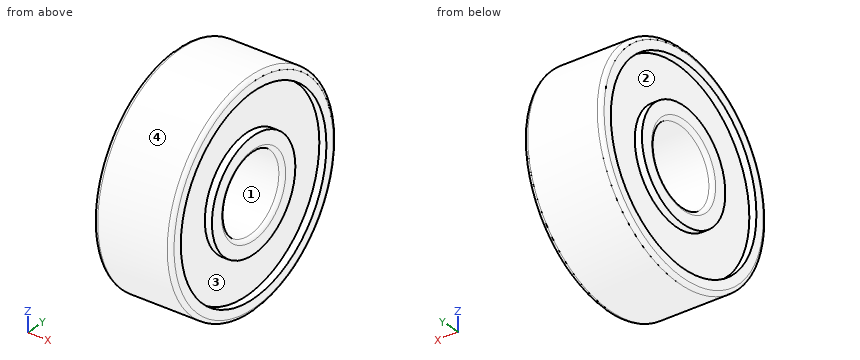
from build123d import *

# Parameters (mm, degrees)
FILLET1_R = 0.3


with BuildPart() as part:
    # Sketch1 → Revolve1 (revolve)
    with BuildSketch(Plane.XY):
        Polygon((0, 3), (6, 3), (6, 4.3), (5.45, 4.3), (5.45, 7.5), (6, 7.5), (6, 8.5), (0, 8.5), (0, 7.5), (0.55, 7.5), (0.55, 4.3), (0, 4.3), align=None)
    revolve(axis=Axis((0, 0, 0), (1, 0, 0)))

    # Fillet1
    fillet1_edges = [part.edges().sort_by_distance(p)[0] for p in [
        (0, -8.5, 0),
        (6, -8.5, 0),
        (6, -3, 0),
        (0, -3, 0),
    ]]
    fillet(fillet1_edges, radius=FILLET1_R)


solid = part.part
CAD build for the part. Positions are in the model's coordinates, mm. Face numbers are marked on the shaded views. A direction names the side the tool comes from. Give positions to 0.01 mm unless a question says otherwise; leave off trailing zeros. Write each loop counter-clockwise with the first axis right and the second up, starting at its lowest first coordinate (ties: lowest second). Pieces come first, ordered by that corner, then holes. Notation, with made-up numbers: (42.5, -37.5) -> (88.5, -37.5) arc R12 cw to (88.5, -18.5) -> close; hole circle Ø11 at (29, 55). An arc over 180 degrees is marked (long way). Return JSON: item names as keys, results as strings.
Item 1: Tool access for the marked faces 1 and 2: list every direction of +Z, -Z, +X, -X, +Y, -Y with a clear straight run to the whole face (end or side of a thin tool).
Answer below:
{"face 1": "+X, -X", "face 2": "-X"}
Item 2: Drill centre lines: probe 1 along Z at (x, y) = (5.6, 0); probe 2 along Z at (x, y) = (2.6, 0); probe 3 along Y at (x, z) = (5.5, 2). Where is each one in solid material? Low to high.
Answer below:
{"probe 1": "z = -8.5 to -7.5, -4.3 to -3, 3 to 4.3, 7.5 to 8.5", "probe 2": "z = -8.5 to -3, 3 to 8.5", "probe 3": "y = -8.26 to -7.23, -3.81 to -2.24, 2.24 to 3.81, 7.23 to 8.26"}
Item 3: Two-plate mould, pull along Z, no slides. Class the marked faces 3 and 4: +Z half, -Z half, draft (parallel to the pull), parting line (faces both ways), or undercut.
Answer below:
{"face 3": "undercut", "face 4": "parting line"}
Item 4: Drop flat-ended pins along their axis: pin 1 (2 mm diameter, centred on x = 2, y = 4, fed in from +Z); pin 2 (2 mm diameter, centred on x = 2.5, y = 2.5, fed in from -Z). Give the stop position or say it passes through.
Answer below:
{"pin 1": "stops at z = 7.95", "pin 2": "stops at z = -8.37"}
Item 5: Band-saw the part on C-C (x = 1.25). List the corners of the cut face in (y, z).
Answer below:
{"outline": "circle Ø17 at (0, 0); hole circle Ø6 at (0, 0)"}
